The figure shows three views and two pictorial views of one solid part (mm, origin at its lowest corner). Answer the questions. A direction names the side the tool comes from. Give positions to 0.01 mm unless a question says otherwise; leave off trailing zeros. Loops run counter-clockwise (first coordinate to the right, second up) from the corner with the lowest first, then second, coordinate; pieces in that order, holes last. Notation, with made-up numbers: M 30,48 L 73,48 A29 cw 73,85 Z; hole C 43.5,19 d3. An arc over 180 degrees is marked long. One line per item, written item: value. Start each with the question number.
Q1. Flat-ended cylindrical pins translate along their axes: pin 1 (4 mm diameter, centred on y = 9.5, z = 27, fed in from +X); pin 2 (3 mm diameter, centred on y = 2, z = 29, fed in from -X). Find the tip coordinate at first contact, or state that the pin passes through.
Q2. A cutting plane is placed at A-A, the plane y = 1.5. Determine the outline of the cut face in (x, z) (1 decimal).
Q3. A cutting plane is placed at B-B, the plane z = 24. Determine the outline of the cut face in (x, y).
Q4. The mould has two halves that part along X. Classify the marked faces 3, 4 and 5: +X half, -X half, draft (parallel to the pull), parting line (faces both ways), or undercut.
Q5. Consider L1, parallel to X at y = 4.5, z = 27; L2, parallel to Y at x = 28, z = 23.5; L3, parallel to Z at x = 33, y = 5.75. Determine where each line is inside the solid, lowest interval first.
Q6. For the marked faces 1 and 2, determine the directions among +Z, -Z, +X, -X, +Y, -Y from which every point of the face is accessible in a straight line to the end or side of a thin tool.
Q7. A cutting plane is placed at D-D, the plane y = 6.75. Determine the outline of the cut face in (x, z) (1 decimal).
Q8. A cutting plane is placed at C-C, the plane x = 18.5. Determine the outline of the cut face in (y, z), and give its area (3 significant figures).
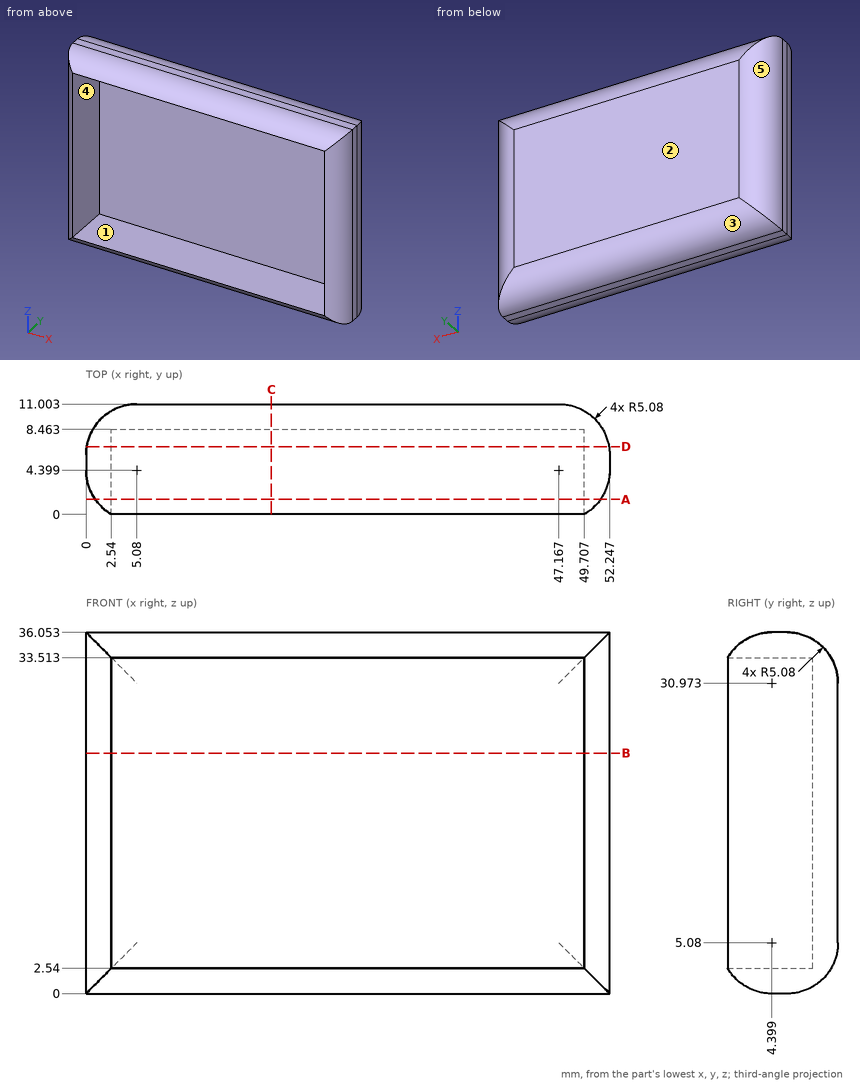
Answer block:
1. pin 1: x = 52
1. pin 2: x = 0.08
2. outline: M 0.9,0.9 L 51.3,0.9 L 51.3,35.1 L 0.9,35.1 Z; hole M 2.5,2.5 L 49.7,2.5 L 49.7,33.5 L 2.5,33.5 Z
3. outline: M 0,4.4 A5.08 ccw 2.54,0 L 2.54,8.46 L 49.71,8.46 L 49.71,0 A5.08 ccw 52.25,4.4 L 52.25,5.92 A5.08 ccw 47.17,11 L 5.08,11 A5.08 ccw 0,5.92 Z
4. face 3: draft
4. face 4: undercut
4. face 5: -X half
5. L1: 0 to 2.54, 49.71 to 52.25
5. L2: 8.46 to 11
5. L3: 0 to 2.54, 33.51 to 36.05
6. face 1: -Y
6. face 2: +Z, -Z, +X, -X, +Y
7. outline: M 0.1,0.1 L 52.2,0.1 L 52.2,36 L 0.1,36 Z; hole M 2.5,2.5 L 49.7,2.5 L 49.7,33.5 L 2.5,33.5 Z
8. outline: M 0,2.54 A5.08 ccw 4.4,0 L 5.92,0 A5.08 ccw 11,5.08 L 11,30.97 A5.08 ccw 5.92,36.05 L 4.4,36.05 A5.08 ccw 0,33.51 L 8.46,33.51 L 8.46,2.54 Z
8. area: 117 mm^2
